from build123d import *

# Parameters (mm, degrees)
SKETCH001_R     = 3
POCKET_DEPTH    = 10
FILLET_R        = 1
FILLET001_R     = 1
SKETCH002_W     = 10
SKETCH002_H     = 5
POCKET001_DEPTH = 28


with BuildPart() as part:
    # Sketch → Revolution (revolve)
    with BuildSketch(Plane.XZ):
        Polygon((-2.2, 0), (-6, 0), (-6, 4), (-4, 4), (-4, 62), (0, 62), (0, 2), (-2.2, 2), align=None)
    revolve(axis=Axis((0, 0, 0), (0, 0, 1)))

    # Sketch001 (on Face5 of Revolution) → Pocket (cut)
    with BuildSketch(Plane(origin=(0, 0, 62), x_dir=(-1, 0, 0), z_dir=(0, 0, 1))):
        Circle(SKETCH001_R)
    extrude(amount=-POCKET_DEPTH, mode=Mode.SUBTRACT)

    # Fillet
    fillet_edges = [part.edges().sort_by_distance(p)[0] for p in [
        (2.2, 0, 0),
        (6, 0, 0),
    ]]
    fillet(fillet_edges, radius=FILLET_R)

    # Fillet001
    fillet001_edges = [part.edges().sort_by_distance(p)[0] for p in [
        (6, 0, 4),
    ]]
    fillet(fillet001_edges, radius=FILLET001_R)

    # Sketch002 (on Face8 of Fillet001) → Pocket001 (cut)
    with BuildSketch(Plane(origin=(0, 0, 62), x_dir=(-1, 0, 0), z_dir=(0, 0, 1))):
        with Locations((0, -6)):
            Rectangle(SKETCH002_W, SKETCH002_H)
        with Locations((0, 6)):
            Rectangle(SKETCH002_W, SKETCH002_H)
    extrude(amount=-POCKET001_DEPTH, mode=Mode.SUBTRACT)


solid = part.part
Part model, mm, in its own coordinate system. A direction names the side the tool comes from. Coordinates: 2 decimals unless noted, no trailing zeros. Loops run counter-clockwise (first coordinate to the right, second up) from the corner with the lowest first, then second, coordinate; pieces in that order, holes last. Notation, with made-up numbers: (73.25, -26) - (94.25, -26) arc R13 ccw to (94.25, -16) - close; hole circle Ø1 at (-15, 32). An arc over 180 degrees is marked (long way). Write each question's results on one line, items separated by ' | '. Start each with the question number.
Q1. Slice it at B-B on z = 56. Give the cut face in (x, y).
Q2. Slice it at C-C on x = 0. Give the cut face in (y, z), and give its area (3 significant figures).
Q3. Slice it at D-D on z = 25.5. Give the cut face in (x, y).
Q4. Slice it at A-A on y = 0. Give the cut face in (x, z).
Q5. Which spindle directions (+Z, -Z, +X, -X, +Y, -Y) get a long thin tool onto all of the face, cutting with end or side? Do faces 1 (the flat face through (0, -3.5, 48)), 2 (the flat face through (0, 0, 52)), 3 (the flat face through (0, 3.5, 48)). Say none if no direction does.
Q6. Probe line 1 along X through (y, z) = (0, 55.5); line 2 along Y through (x, z) = (0, 59); line 3 along Y through (x, z) = (0, 1.7). List the from-to ranges inside material, lowest first.
Q7. Drop flat-ended pins along their axis: pin 1 Ø1.9 at (x, z) = (-1, 43) entering from +Y; pin 2 Ø3 at (y, z) = (-0.5, 48.5) entering from -X; pin 3 Ø5.5 at (x, y) = (0, 0) entering from -Z. Give the stop position or say it passes through.
Q8. Two-plate mould, pull along X, no slides. Class faces 4 (the cylindrical face through (3, 0, 57)), 5 (the cylindrical face through (0.521, -3.966, 33.406)), 6 (the flat face through (3.3, 1, 0)): +X half, -X half, draft (parallel to the pull), parting line (faces both ways), or undercut.
Answer:
1) outline: (-1.94, -3.5) - (1.94, -3.5) arc R4 ccw to (1.94, 3.5) - (-1.94, 3.5) arc R4 ccw to start; hole circle Ø6 at (0, 0)
2) outline: (-6, 1) arc R1 ccw to (-5, 0) - (-3.2, 0) arc R1 ccw to (-2.2, 1) - (-2.2, 2) - (2.2, 2) - (2.2, 1) arc R1 ccw to (3.2, 0) - (5, 0) arc R1 ccw to (6, 1) - (6, 3) arc R1 ccw to (5, 4) - (4, 4) - (4, 34) - (3.5, 34) - (3.5, 62) - (3, 62) - (3, 52) - (-3, 52) - (-3, 62) - (-3.5, 62) - (-3.5, 34) - (-4, 34) - (-4, 4) - (-5, 4) arc R1 ccw to (-6, 3) - close | area: 414 mm2
3) outline: circle Ø8 at (0, 0)
4) outline: (-6, 1) arc R1 ccw to (-5, 0) - (-3.2, 0) arc R1 ccw to (-2.2, 1) - (-2.2, 2) - (2.2, 2) - (2.2, 1) arc R1 ccw to (3.2, 0) - (5, 0) arc R1 ccw to (6, 1) - (6, 3) arc R1 ccw to (5, 4) - (4, 4) - (4, 62) - (3, 62) - (3, 52) - (-3, 52) - (-3, 62) - (-4, 62) - (-4, 4) - (-5, 4) arc R1 ccw to (-6, 3) - close
5) face 1: +Z, +X, -X, -Y | face 2: +Z | face 3: +Z, +X, -X, +Y
6) line 1: x = -4 to -3, 3 to 4 | line 2: y = -3.5 to -3, 3 to 3.5 | line 3: y = -6 to -2.2, 2.2 to 6
7) pin 1: stops at y = 3.5 | pin 2: stops at x = -4 | pin 3: stops at z = 0.11
8) face 4: undercut | face 5: parting line | face 6: draft
